Check sheet for the modelled part. Datum: model origin and axes. Units: mm. A direction names the side the tool comes from. Round coordinates to 2 decimals unless told otherwise and drop trailing zeros. Loops run counter-clockwise (first coordinate to the right, second up) from the corner with the lowest first, then second, coordinate; pieces in that order, holes last. Notation, with made-up numbers: (35, -39) -> (65, -39) arc R33 ccw to (65, -11) -> close; hole circle Ø7 at (75, 50.25). An arc over 180 degrees is marked (long way). Return JSON: item names as keys, results as strings.
from build123d import *

# Parameters (mm, degrees)
SKETCH1_R           = 50
BOSS_EXTRUDE1_DEPTH = 5
SKETCH2_R           = 41.5
BOSS_EXTRUDE2_DEPTH = 20
SKETCH4_W           = 4
SKETCH4_H           = 2
SKETCH6_R           = 30
CUT_EXTRUDE1_DEPTH  = 76


with BuildPart() as part:
    # Sketch1 → Boss-Extrude1 (new body)
    with BuildSketch(Plane.XY):
        Circle(SKETCH1_R)
    extrude(amount=BOSS_EXTRUDE1_DEPTH)

    # Sketch2 → Boss-Extrude2 (add)
    with BuildSketch(Plane.XY.offset(5)):
        Circle(SKETCH2_R)
    extrude(amount=BOSS_EXTRUDE2_DEPTH)

    # Sketch4 → Cut-Revolve1 (revolve, cut)
    with BuildSketch(Plane(origin=(0, 0, 0), x_dir=(0, 0, -1), z_dir=(1, 0, 0))):
        with Locations((-11, 40.5)):
            Rectangle(SKETCH4_W, SKETCH4_H)
        with Locations((-19, 40.5)):
            Rectangle(SKETCH4_W, SKETCH4_H)
    revolve(axis=Axis((0, 0, 0), (0, 0, 1)), mode=Mode.SUBTRACT)

    # Sketch6 → Cut-Extrude1 (cut, through all)
    with BuildSketch(Plane.XY.offset(25)):
        Circle(SKETCH6_R)
    extrude(amount=-CUT_EXTRUDE1_DEPTH, mode=Mode.SUBTRACT)

    # Sketch5 → Revolve2 (revolve)
    with BuildSketch(Plane(origin=(0, 0, 0), x_dir=(0, 0, -1), z_dir=(1, 0, 0)), mode=Mode.PRIVATE) as revolve2_sk:
        with BuildLine():
            add(Edge.make_bspline(
                [(60, 0), (60, -30), (18.341729935, -47.585265444), (0, -50)],
                knots=[0, 0, 0, 0, 1, 1, 1, 1], degree=3))
            Line((60, 0), (57, 0))
            add(Edge.make_bspline(
                [(57, 0), (57, -0.839529251), (56.926216151, -2.532697799), (56.498585906, -5.787348513), (55.464384581, -9.710785416), (53.492757525, -14.183558613), (49.97819358, -19.848130616), (44.10315688, -26.337560331), (35.370011046, -33.045053917), (27.328482154, -37.640390457), (20.829690882, -40.681617372), (16.022193995, -42.637477595), (11.381613041, -44.261311839), (7.738449227, -45.332702164), (5.011819594, -46.017990599), (3.073688428, -46.445655401), (1.563551079, -46.729287857), (0.591183995, -46.88571964), (0.174241223, -46.947356625), (0.033004859, -46.967504681), (0, -46.972173716)],
                knots=[0, 0, 0, 0, 0.03125, 0.0625, 0.125, 0.1875, 0.25, 0.375, 0.5, 0.625, 0.6875, 0.75, 0.8125, 0.875, 0.90625, 0.9375, 0.96875, 0.984375, 0.990544401, 0.99243552, 0.99243552, 0.99243552, 0.99243552], degree=3))
            Line((0, -46.972173716), (0, -50))
        make_face()
    revolve(revolve2_sk.sketch.rotate(Axis((0, 0, 0), (0, 0, -1)), 180), axis=Axis((0, 0, 0), (0, 0, -1)))


solid = part.part
Q1. Go/stop test with flat-tipped pins: pin 1 (1.5 mm diameter, centred on y = -35.5, z = -40, fed in from +X); pin 2 (12 mm diameter, centred on x = 26.5, y = -19, fed in from -Z); pin 3 (3 mm diameter, centred on x = 10, y = -11.5, fed in from -Z); pin 4 (5 mm diameter, centred on y = 13.5, z = -45.5, fed in from -X). Record where each tip stops, or that it passes through.
Results list:
{"pin 1": "through", "pin 2": "z = -47.69", "pin 3": "z = -56.93", "pin 4": "x = -28.01"}
Q2. Section check A-A (z = 18.5). Record the boundary of the cut face in (x, y).
Results list:
{"outline": "circle Ø79 at (0, 0); hole circle Ø60 at (0, 0)"}
Q3. Tool access check on faces 1 (the cylindrical face through (-26.7, -29.11, 18.97)), 2 (the cylindrical face through (38.335, -15.895, 14.972)), 3 (the cylindrical face through (47.69, 15.02, 2.46)). Record the directions out of +Z, -Z, +X, -X, +Y, -Y that give a thin tool (end or side, any length) a straight path to the whole face; none if there is none.
Results list:
{"face 1": "none", "face 2": "+Z", "face 3": "+Z, -Z"}
Q4. Material ranges on line 1 (Y direction, x = 0, z = 10); line 2 (Y direction, x = 0, z = 7); line 3 (Z direction, x = -24.5, y = -18.5), recorded low to high.
Results list:
{"line 1": "-39.5 to -30, 30 to 39.5", "line 2": "-41.5 to -30, 30 to 41.5", "line 3": "-43.17 to -38.28, 0 to 25"}
Q5. Draft check along X on faces 4 (the flat face through (-18.8, 37.3, 5)), 5 (the flat face through (-1, -31, 0)), 6 (the cylindrical face through (38.335, -15.895, 6.972)), 7 (the cylindrical face through (-29.97, 1.32, 12.68)). Enter one of: released by +X, released by -X, zero draft, split by the parting line, or undercut.
Results list:
{"face 4": "zero draft", "face 5": "undercut", "face 6": "split by the parting line", "face 7": "undercut"}
